Input: part model. Units: mm. Frame: model coordinates. A direction names the side the tool comes from. Give positions to 0.01 mm unless a question says otherwise; leave off trailing zeros. Loops run counter-clockwise (first coordinate to the right, second up) from the corner with the lowest first, then second, coordinate; pieces in that order, holes last. Notation, with made-up numbers: M 89.5,9.25 L 132.5,9.25 A37 cw 132.5,48.25 Z; hole C 48.25,62.5 d1. An arc over 180 degrees is marked long. Use a Markdown table: item, result. Add a question column.
from build123d import *
from build123d.topology import SkipClean

# Parameters (mm, degrees)
SKETCH1_W                       = 80
SKETCH1_H                       = 12
BOSS_EXTRUDE1_DEPTH             = 2
CUT_REVOLVE1_ANGLE              = 180
FILLET2_R                       = 4
BOSS_EXTRUDE2_REACH             = 42.645
SKETCH6_R                       = 17
BOSS_EXTRUDE2_DIRECTION_2_DEPTH = 2
SKETCH7_R                       = 2.5
CUT_EXTRUDE3_DEPTH              = 3
CIRPATTERN1_COUNT               = 6
FILLET3_R                       = 1
CUT_EXTRUDE4_REACH              = 61.783
SKETCH8_R                       = 1.5
CUT_EXTRUDE5_REACH              = 61.783
SKETCH9_R                       = 1.5


with BuildPart() as part:
    # Sketch1 → Boss-Extrude1 (new, symmetric)
    with BuildSketch(Plane.XY):
        Rectangle(SKETCH1_W, SKETCH1_H)
    extrude(amount=BOSS_EXTRUDE1_DEPTH, both=True)

    # Sketch3 → Cut-Revolve1 (revolve, cut)
    with SkipClean():  # the faces are left unmerged after this step: merging them gives an invalid solid
        with BuildSketch(Plane.XY.offset(-2)):
            with BuildLine():
                ThreePointArc((37.75, 0), (35, 2.75), (32.25, 0))
                Line((32.25, 0), (37.75, 0))
            make_face()
            with BuildLine():
                Line((37.75, 0), (32.25, 0))
                ThreePointArc((32.25, 0), (35, -2.75), (37.75, 0))
            make_face()
        revolve(axis=Axis((32.25, 0, -2), (1, 0, 0)), revolution_arc=CUT_REVOLVE1_ANGLE, mode=Mode.SUBTRACT)

    # Fillet2
    fillet2_edges = [part.edges().sort_by_distance(p)[0] for p in [
        (40, -6, 0),
        (40, 6, 0),
    ]]
    fillet(fillet2_edges, radius=FILLET2_R)

    # Boss-Extrude2: up to this face of the body (flat: up to its plane)
    boss_extrude2_end = Plane(part.part.faces().sort_by_distance((-1.183693998, 0, -2))[0])
    # Sketch6 → Boss-Extrude2 (add, up to the picked face)
    with BuildSketch(Plane.XY.offset(2), mode=Mode.PRIVATE) as boss_extrude2_sk1:
        with Locations(Location((-40, 0, 0), (0, 0, 20.667316494))):
            Circle(SKETCH6_R)
    boss_extrude2_tool1 = split(extrude(boss_extrude2_sk1.sketch, amount=-BOSS_EXTRUDE2_REACH, mode=Mode.PRIVATE), bisect_by=boss_extrude2_end, keep=Keep.BOTH, mode=Mode.PRIVATE)
    add(boss_extrude2_tool1.solids().sort_by(Axis((-40, 0, 2), (0, 0, -1)))[0])

    # Sketch6 → Boss-Extrude2 direction 2 (add)
    with BuildSketch(Plane.XY.offset(2)):
        with Locations(Location((-40, 0, 0), (0, 0, 20.667316494))):
            Circle(SKETCH6_R)
    extrude(amount=BOSS_EXTRUDE2_DIRECTION_2_DEPTH)

    # Sketch7 → Cut-Extrude3 (cut)
    with BuildSketch(Plane(origin=(0, 0, -2), x_dir=(-1, 0, 0), z_dir=(0, 0, -1))):
        with BuildLine():
            Line((41.148365434, 4.169758006), (40, 4.325))
            ThreePointArc((40, 4.325), (35.675, 0), (40, -4.325))
            Line((40, -4.325), (41.148365434, -4.169758006))
            ThreePointArc((41.148365434, -4.169758006), (43.440371019, -2.620967808), (44.325, 0))
            ThreePointArc((44.325, 0), (43.440371019, 2.620967808), (41.148365434, 4.169758006))
        make_face()
        with BuildLine():
            Line((53.5, 2.5), (41.148365434, 4.169758006))
            ThreePointArc((41.148365434, 4.169758006), (43.440371019, 2.620967808), (44.325, 0))
            ThreePointArc((44.325, 0), (43.440371019, -2.620967808), (41.148365434, -4.169758006))
            Line((41.148365434, -4.169758006), (53.5, -2.5))
            ThreePointArc((53.5, -2.5), (51, 0), (53.5, 2.5))
        make_face()
        with Locations((53.5, 0)):
            Circle(SKETCH7_R)
    cut_extrude3 = extrude(amount=-CUT_EXTRUDE3_DEPTH, mode=Mode.SUBTRACT)

    # CirPattern1: Cut-Extrude3 ×6 about axis
    cirpattern1_axis = Axis((-40, 0, 0), (0, 0, 1))
    for i in range(1, CIRPATTERN1_COUNT):
        add(cut_extrude3.rotate(cirpattern1_axis, i * 360 / CIRPATTERN1_COUNT), mode=Mode.SUBTRACT)

    # Fillet3
    fillet3_edges = [part.edges().sort_by_distance(p)[0] for p in [
        (-46.069873399, 3.504443041, -0.5),
        (-40, 7.008886081, -0.5),
        (-33.930126601, 3.504443041, -0.5),
        (-33.930126601, -3.504443041, -0.5),
        (-40, -7.008886081, -0.5),
        (-46.069873399, -3.504443041, -0.5),
    ]]
    fillet(fillet3_edges, radius=FILLET3_R)

    # Sketch8 → Cut-Extrude4 (cut, up to next)
    with BuildSketch(Plane.XY.offset(4), mode=Mode.PRIVATE) as cut_extrude4_sk1:
        with Locations((-40, 0)):
            Circle(SKETCH8_R)
    cut_extrude4_tool1 = extrude(cut_extrude4_sk1.sketch, amount=-CUT_EXTRUDE4_REACH, mode=Mode.PRIVATE) & part.part
    add(cut_extrude4_tool1.solids().sort_by_distance((-40, 0, 4))[0], mode=Mode.SUBTRACT)

    # Sketch9 → Cut-Extrude5 (cut, up to next)
    with BuildSketch(Plane(origin=(0, 0, -2), x_dir=(-1, 0, 0), z_dir=(0, 0, -1)), mode=Mode.PRIVATE) as cut_extrude5_sk1:
        with Locations((2.5, 0)):
            Circle(SKETCH9_R)
    cut_extrude5_tool1 = extrude(cut_extrude5_sk1.sketch, amount=-CUT_EXTRUDE5_REACH, mode=Mode.PRIVATE) & part.part
    add(cut_extrude5_tool1.solids().sort_by_distance((-2.5, 0, -2))[0], mode=Mode.SUBTRACT)


solid = part.part
1) Pull-direction query (X, two-part tool) for faces 3 (the cylindrical face through (-56, 0, -1)), 4 (the cylindrical face through (38.797, 4.859, -0.028)), 5 (the flat face through (-47.72, 7.53, -0.52)), 6 (the flat face through (-20, 0, -2)); classes: pulls with the +X half, pulls with the -X half, needs draft (parallel to the pull), parting line crosses it, or undercut.
2) Section query A-A, the plane x = -2.5. Return the cut outline in (y, z).
3) Section query B-B, the plane z = -1.05. State how many separate pieces and enclosed holes the cut face has, and give its area (3 significant figures).
4) Contact query for flat-ended pins moving along their axis: P1, Ø0.5, axis at x = -44, y = 2, coming from the -Z side; P2, Ø2, axis at y = -9, z = -1.5, coming from the +X side; P3, Ø1.8, axis at x = -40, y = 0, coming from the +Z side; P4, Ø2, axis at x = 15.5, z = 0.5, coming from the +Y side. Output: stop coordinate, or through.
5) Ray query, line 1 (Y direction, x = -2.5, z = 1.1); line 2 (X direction, y = 9.5, z = -1.2); line 3 (X direction, y = -12, z = 0.25). Return the intervals inside material, ascending. Write a range as [from, to].
6) Reachability of faces 1 (the flat face through (-32.28, -7.53, -0.52)), 2 (the flat face through (40, 0, 0)) from +Z, -Z, +X, -X, +Y, -Y: full face, straight path, thin tool, end or side. Return the list, or none.
Entries:
| question | item | result |
|---|---|---|
| 1 | face 3 | undercut |
| 1 | face 4 | pulls with the +X half |
| 1 | face 5 | undercut |
| 1 | face 6 | needs draft |
| 2 | outline | M -6,-2 L -1.5,-2 L -1.5,2 L -6,2 Z; M 1.5,-2 L 6,-2 L 6,2 L 1.5,2 Z |
| 3 | separate pieces | 1 |
| 3 | enclosed holes | 3 |
| 3 | area | 1,180 mm² |
| 4 | P1 | stops at z = 1 |
| 4 | P2 | stops at x = -25 |
| 4 | P3 | passes through |
| 4 | P4 | stops at y = 6 |
| 5 | line 1 | y = [-6, -1.5], [1.5, 6] |
| 5 | line 2 | x = [-54.1, -48.53], [-41.93, -38.07], [-31.47, -25.9] |
| 5 | line 3 | x = [-52.04, -49.23], [-43.86, -36.14], [-30.77, -27.96] |
| 6 | face 1 | -Z |
| 6 | face 2 | +Z, -Z, +X, +Y, -Y |
